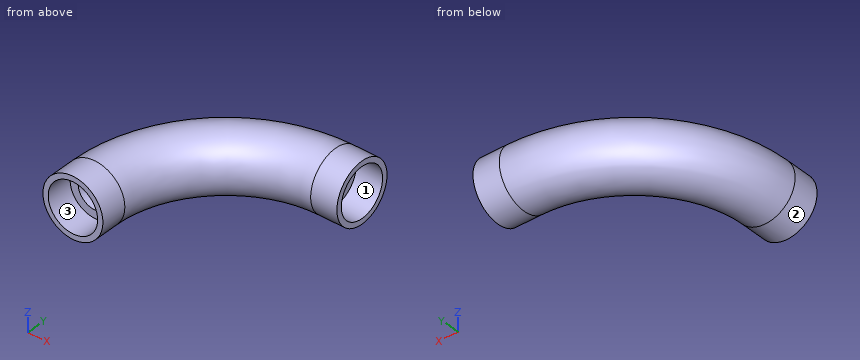
```python
from build123d import *

# Parameters (mm, degrees)
F1_R     = 5.715
F1_R_2   = 3.175
F3_R     = 5.715
F3_R_2   = 4.70576
F4_DEPTH = 5
F5_R     = 5.715
F5_R_2   = 4.70576
F6_DEPTH = 5


with BuildPart() as f2:
    # F2: sweep along a path in F0
    with BuildLine(Plane.XY) as f2_path:
        ThreePointArc((-25, 0), (-17.6776695297, 17.6776695297), (0, 25))
    # F1 (on Front) → F2 (sweep)
    with BuildSketch(Plane.XZ):
        with Locations((-25, 0)):
            Circle(F1_R)
        with Locations((-25, 0)):
            Circle(F1_R_2, mode=Mode.SUBTRACT)
    sweep(path=f2_path.line)

    # F3 (on face) → F4 (join)
    with BuildSketch(Plane.XZ):
        with Locations((-25, 0)):
            Circle(F3_R)
        with Locations((-25, 0)):
            Circle(F3_R_2, mode=Mode.SUBTRACT)
    extrude(amount=F4_DEPTH)

    # F5 (on face) → F6 (join)
    with BuildSketch(Plane.YZ):
        with Locations((25, 0)):
            Circle(F5_R)
        with Locations((25, 0)):
            Circle(F5_R_2, mode=Mode.SUBTRACT)
    extrude(amount=F6_DEPTH)


solid = f2.part
```
Geometry check sheet. Reference: the model listing, model coordinates, mm. Face numbers are marked on the shaded views. Coordinates: 2 decimals unless noted, no trailing zeros. Order: outer loops, then holes, each group sorted by start corner. A loop starts at its lowest first (then second) coordinate and runs counter-clockwise, first axis right, second up.
Q1. Depth check by flat-ended pin: pin 1 Ø1 at (x, z) = (-1, -4) entering from +Y; pin 2 Ø2 at (x, z) = (-26.5, 2.5) entering from +Y; pin 3 Ø1.5 at (y, z) = (21, -2) entering from -X. Enter the tip coordinate at first touch or a pass-through.
Reply:
pin 1: stops at y = 29.5
pin 2: stops at y = 16.26
pin 3: stops at x = -22.69
Q2. Sectioned sample at A-A on z = 2.75. Record the cut outline in (x, y).
Reply:
outline: (-30.01, -5) - (-28.82, -5) - (-28.82, 0) - (-26.59, 0) arc R26.59 cw to (0, 26.59) - (0, 28.82) - (5, 28.82) - (5, 30.01) - (0, 30.01) arc R30.01 ccw to (-30.01, 0) - close; (-23.41, 0) - (-21.18, 0) - (-21.18, -5) - (-19.99, -5) - (-19.99, 0) arc R19.99 cw to (0, 19.99) - (5, 19.99) - (5, 21.18) - (0, 21.18) - (0, 23.41) arc R23.41 ccw to start
Q3. Sectioned sample at D-D on z = -1.5. Record the cut outline in (x, y), and give its area (3 significant figures).
Reply:
outline: (-30.51, -5) - (-29.46, -5) - (-29.46, 0) - (-27.8, 0) arc R27.8 cw to (0, 27.8) - (0, 29.46) - (5, 29.46) - (5, 30.51) - (0, 30.51) arc R30.51 ccw to (-30.51, 0) - close; (-22.2, 0) - (-20.54, 0) - (-20.54, -5) - (-19.49, -5) - (-19.49, 0) arc R19.49 cw to (0, 19.49) - (5, 19.49) - (5, 20.54) - (0, 20.54) - (0, 22.2) arc R22.2 ccw to start
area: 234 mm2
Q4. Draft check along Z on the marked faces 1, 2 and 3. Enter one of: released by +Z, released by -Z, zero draft, split by the parting line, or undercut.
Reply:
face 1: undercut
face 2: split by the parting line
face 3: undercut
Q5. Thickness scan on probe 1 along Z at (x, y) = (-25, -1) (3 decimals); probe 2 along Y at (x, z) = (-13, -2.5); probe 3 along Y at (x, z) = (-4, 0.5). Record the ranges inside material, lowest first.
Reply:
probe 1: z = -5.715 to -4.706, 4.706 to 5.715
probe 2: y = 15.02 to 19.03, 23.62 to 27.19
probe 3: y = 18.89 to 21.5, 27.85 to 30.43
Q6. Sectioned sample at C-C on x = 2. Record the cut outline in (y, z) (3 decimals), and give its area (3 significant figures).
Reply:
outline: circle Ø11.43 at (25, 0); hole circle Ø9.412 at (25, 0)
area: 33.0 mm2
Q7. Sectioned sample at B-B on z = -4.25. Record the cut outline in (x, y), and give its area (3 significant figures).
Reply:
outline: (-28.82, -5) - (-27.02, -5) - (-27.02, 0) - (-22.98, 0) - (-22.98, -5) - (-21.18, -5) - (-21.18, 0) arc R21.18 cw to (0, 21.18) - (5, 21.18) - (5, 22.98) - (0, 22.98) - (0, 27.02) - (5, 27.02) - (5, 28.82) - (0, 28.82) arc R28.82 ccw to (-28.82, 0) - close
area: 336 mm2
